Can you work these out from the model? Positions are in its coordinate system, mm. Face numbers are marked on the shaded views. A direction names the side the tool comes from. Give positions to 0.01 mm unless a question says otherwise; leave off trailing zeros. Order: outer loops, then holes, each group sorted by start corner. A loop starts at its lowest first (then second) coordinate and runs counter-clockwise, first axis right, second up. Notation, with made-up numbers: M -18,76.25 L 30,76.25 A35 ccw 30,109.25 Z; hole C 7,61 d4. An arc over 180 degrees is marked long. One line per question, with ' | ' between items. Start each with the question number.
1) If we section it at A-A, the plane z = -57: Please give me the cut outline in (x, y) (3 decimals).
2) For the marked faces 1 and 2, which set-ups out of +Z, -Z, +X, -X, +Y, -Y let a thin tool reach every point of the face, with its end or its side?
3) If we section it at C-C, the plane x = 33: Please give me the cut outline in (y, z) (3 decimals), plus the area to 3 significant figures.
4) Please list where these lines run through material, in increasing order: line 1 along X through (y, z) = (-46, -16); line 2 along Y through (x, z) = (29.5, -2) (3 decimals); line 3 along Z through (x, y) = (55.5, -19.5). Write a range as [from, to].
5) If we section it at B-B, the plane y = 160: Please give me the cut outline in (x, z).
6) If we section it at D-D, the plane y = -24: Please give me the cut outline in (x, z), plus the area to 3 significant figures.
7) I'm going to push flat-ended pins straight in: pin 1 Ø2 at (x, y) = (47.5, 255.5) entering from +Z; pin 2 Ø0.8 at (x, z) = (-48.5, -83) entering from -Y (3 decimals); pin 3 Ø10 at (y, z) = (-34.5, -48) entering from +X; pin 4 Ø1.2 at (x, z) = (-48, -7) entering from +Y (3 decimals). Where does each tip first touch, or does it pass through?
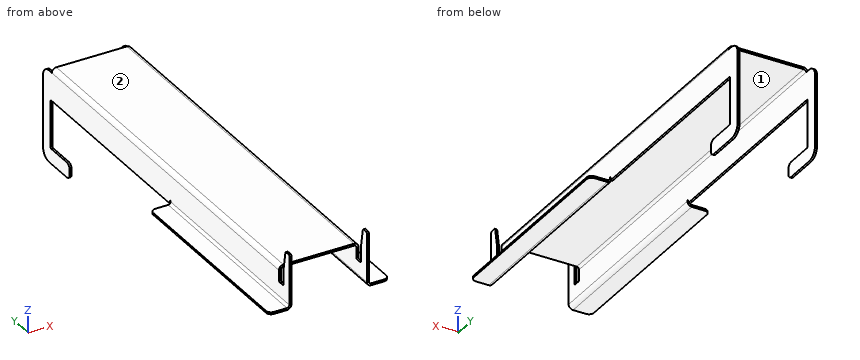
```python
from build123d import *

# Parameters (mm, degrees)
SKETCH1_W                     = 99.06
SKETCH1_H                     = 508
BASE_FLANGE1_DEPTH            = 2.5
EDGE_FLANGE1_STRIP_W          = 16
EDGE_FLANGE1_STRIP_H          = 2.5
EDGE_FLANGE1_STRIP_CUT_DEPTH  = 508
EDGE_FLANGE1_DEPTH            = 508
EDGE_FLANGE2_STRIP_W          = 16
EDGE_FLANGE2_STRIP_H          = 2.5
EDGE_FLANGE2_STRIP_CUT_DEPTH  = 254
EDGE_FLANGE2_RELIEF_W         = 17.25
EDGE_FLANGE2_RELIEF_H         = 1.25
EDGE_FLANGE2_RELIEF_CUT_DEPTH = 2.5
EDGE_FLANGE2_DEPTH            = 254
EDGE_FLANGE2_START            = 2.5
EDGE_FLANGE2_FLAT_DEPTH       = 2.5
EDGE_FLANGE3_STRIP_W          = 16
EDGE_FLANGE3_STRIP_H          = 2.5
EDGE_FLANGE3_STRIP_CUT_DEPTH  = 508
EDGE_FLANGE3_DEPTH            = 508
EDGE_FLANGE4_STRIP_W          = 16
EDGE_FLANGE4_STRIP_H          = 2.5
EDGE_FLANGE4_STRIP_CUT_DEPTH  = 254
EDGE_FLANGE4_RELIEF_W         = 17.25
EDGE_FLANGE4_RELIEF_H         = 1.25
EDGE_FLANGE4_RELIEF_CUT_DEPTH = 2.5
EDGE_FLANGE4_DEPTH            = 254
EDGE_FLANGE4_START            = 2.5
EDGE_FLANGE4_FLAT_DEPTH       = 2.5
SKETCH22_W                    = 5.5
SKETCH22_H                    = 22.225
CUT_EXTRUDE5_DEPTH            = 287.118684465
TAB1_DEPTH                    = 2.5
TAB2_START                    = -2.5
TAB2_DEPTH                    = 2.5
TAB3_DEPTH                    = 2.5
TAB4_START                    = -2.5
TAB4_DEPTH                    = 2.5
SKETCH47_W                    = 14.2875
SKETCH47_H                    = 9.525
CUT_EXTRUDE6_DEPTH            = 337.63035334
FILLET2_R                     = 1.5875
FILLET3_R                     = 1.5875
SKETCH48_W                    = 2.54
SKETCH48_H                    = 15.875
CUT_EXTRUDE9_DEPTH            = 337.63035334
FILLET4_R                     = 12.7


# Read off the part's stored shape, not the designer's step: Tab2
# Sheet-metal steps are written as plain solids
with BuildPart() as part:
    # Sketch1 → Base-Flange1 (new body)
    with BuildSketch(Plane.XY):
        Rectangle(SKETCH1_W, SKETCH1_H)
    extrude(amount=-BASE_FLANGE1_DEPTH)

    # Edge-Flange1 strip (across the edge) → Edge-Flange1 strip cut (cut)
    with BuildSketch(Plane(origin=(-49.53, -254, -2.5), x_dir=(1, 0, 0), z_dir=(0, 1, 0))):
        with Locations((-2.5, -1.25)):
            Rectangle(EDGE_FLANGE1_STRIP_W, EDGE_FLANGE1_STRIP_H)
    extrude(amount=EDGE_FLANGE1_STRIP_CUT_DEPTH, mode=Mode.SUBTRACT)

    # Edge-Flange1 section (across the edge) → Edge-Flange1 (add)
    with BuildSketch(Plane(origin=(-49.53, -254, -2.5), x_dir=(1, 0, 0), z_dir=(0, 1, 0))):
        with BuildLine():
            Line((0, 3), (0, 38.1))
            Line((0, 38.1), (2.5, 38.1))
            Line((2.5, 38.1), (2.5, 3))
            ThreePointArc((2.5, 3), (3.378679656, 0.878679656), (5.5, 0))
            Line((5.5, 0), (5.5, -2.5))
            ThreePointArc((5.5, -2.5), (1.610912703, -0.889087297), (0, 3))
        make_face()
    extrude(amount=EDGE_FLANGE1_DEPTH)

    # Edge-Flange2 strip (across the edge) → Edge-Flange2 strip cut (cut)
    with BuildSketch(Plane(origin=(-49.53, 0, -40.6), x_dir=(0, 0, 1), z_dir=(0, -1, 0))):
        with Locations((-5, -1.25)):
            Rectangle(EDGE_FLANGE2_STRIP_W, EDGE_FLANGE2_STRIP_H)
    extrude(amount=EDGE_FLANGE2_STRIP_CUT_DEPTH, mode=Mode.SUBTRACT)

    # Edge-Flange2 relief (on the sheet) → Edge-Flange2 relief cut (cut)
    with BuildSketch(Plane(origin=(-49.53, 0, -37.6), x_dir=(0, 0, 1), z_dir=(-1, 0, 0))):
        with Locations((-7.375, 0.625)):
            Rectangle(EDGE_FLANGE2_RELIEF_W, EDGE_FLANGE2_RELIEF_H)
    extrude(amount=-EDGE_FLANGE2_RELIEF_CUT_DEPTH, mode=Mode.SUBTRACT)

    # Edge-Flange2 bend section (across the edge) → Edge-Flange2 (add)
    with BuildSketch(Plane(origin=(-49.53, 0, -40.6), x_dir=(0, 0, 1), z_dir=(0, -1, 0))):
        with BuildLine():
            Line((-2.5, 3), (0, 3))
            ThreePointArc((0, 3), (0.878679656, 0.878679656), (3, 0))
            Line((3, 0), (3, -2.5))
            ThreePointArc((3, -2.5), (-0.889087297, -0.889087297), (-2.5, 3))
        make_face()
    extrude(amount=EDGE_FLANGE2_DEPTH)

    # Edge-Flange2 profile (on flange) → Edge-Flange2 flat (add)
    with BuildSketch(Plane(origin=(-49.53, 0, -40.6), x_dir=(0, -1, 0), z_dir=(0, 0, -1)).offset(EDGE_FLANGE2_START)):
        with BuildLine():
            Line((254, 3), (254, 19.05))
            ThreePointArc((254, 19.05), (252.140128061, 23.540128061), (247.65, 25.4))
            Line((247.65, 25.4), (6.35, 25.4))
            ThreePointArc((6.35, 25.4), (1.859871939, 23.540128061), (0, 19.05))
            Line((0, 19.05), (0, 3))
            Line((0, 3), (254, 3))
        make_face()
    extrude(amount=-EDGE_FLANGE2_FLAT_DEPTH)

    # Edge-Flange3 strip (across the edge) → Edge-Flange3 strip cut (cut)
    with BuildSketch(Plane(origin=(49.53, 254, -2.5), x_dir=(-1, 0, 0), z_dir=(0, -1, 0))):
        with Locations((-2.5, -1.25)):
            Rectangle(EDGE_FLANGE3_STRIP_W, EDGE_FLANGE3_STRIP_H)
    extrude(amount=EDGE_FLANGE3_STRIP_CUT_DEPTH, mode=Mode.SUBTRACT)

    # Edge-Flange3 section (across the edge) → Edge-Flange3 (add)
    with BuildSketch(Plane(origin=(49.53, 254, -2.5), x_dir=(-1, 0, 0), z_dir=(0, -1, 0))):
        with BuildLine():
            Line((0, 3), (0, 38.1))
            Line((0, 38.1), (2.5, 38.1))
            Line((2.5, 38.1), (2.5, 3))
            ThreePointArc((2.5, 3), (3.378679656, 0.878679656), (5.5, 0))
            Line((5.5, 0), (5.5, -2.5))
            ThreePointArc((5.5, -2.5), (1.610912703, -0.889087297), (0, 3))
        make_face()
    extrude(amount=EDGE_FLANGE3_DEPTH)

    # Edge-Flange4 strip (across the edge) → Edge-Flange4 strip cut (cut)
    with BuildSketch(Plane(origin=(49.53, -254, -40.6), x_dir=(0, 0, 1), z_dir=(0, 1, 0))):
        with Locations((-5, -1.25)):
            Rectangle(EDGE_FLANGE4_STRIP_W, EDGE_FLANGE4_STRIP_H)
    extrude(amount=EDGE_FLANGE4_STRIP_CUT_DEPTH, mode=Mode.SUBTRACT)

    # Edge-Flange4 relief (on the sheet) → Edge-Flange4 relief cut (cut)
    with BuildSketch(Plane(origin=(49.53, -254, -37.6), x_dir=(0, 0, 1), z_dir=(1, 0, 0))):
        with Locations((-7.375, -254.625)):
            Rectangle(EDGE_FLANGE4_RELIEF_W, EDGE_FLANGE4_RELIEF_H)
    extrude(amount=-EDGE_FLANGE4_RELIEF_CUT_DEPTH, mode=Mode.SUBTRACT)

    # Edge-Flange4 bend section (across the edge) → Edge-Flange4 (add)
    with BuildSketch(Plane(origin=(49.53, -254, -40.6), x_dir=(0, 0, 1), z_dir=(0, 1, 0))):
        with BuildLine():
            Line((-2.5, 3), (0, 3))
            ThreePointArc((0, 3), (0.878679656, 0.878679656), (3, 0))
            Line((3, 0), (3, -2.5))
            ThreePointArc((3, -2.5), (-0.889087297, -0.889087297), (-2.5, 3))
        make_face()
    extrude(amount=EDGE_FLANGE4_DEPTH)

    # Edge-Flange4 profile (on flange) → Edge-Flange4 flat (add)
    with BuildSketch(Plane(origin=(49.53, 0, -40.6), x_dir=(0, 1, 0), z_dir=(0, 0, -1)).offset(EDGE_FLANGE4_START)):
        with BuildLine():
            Line((-254, 19.05), (-254, 3))
            Line((-254, 3), (0, 3))
            Line((0, 3), (0, 19.05))
            ThreePointArc((0, 19.05), (-1.859871939, 23.540128061), (-6.35, 25.4))
            Line((-6.35, 25.4), (-247.65, 25.4))
            ThreePointArc((-247.65, 25.4), (-252.140128061, 23.540128061), (-254, 19.05))
        make_face()
    extrude(amount=-EDGE_FLANGE4_FLAT_DEPTH)

    # Sketch22 → Cut-Extrude5 (cut, through all)
    with BuildSketch(Plane.ZY.offset(49.53)):
        with Locations((-2.75, -242.8875)):
            Rectangle(SKETCH22_W, SKETCH22_H)
    extrude(amount=-CUT_EXTRUDE5_DEPTH, mode=Mode.SUBTRACT)

    # Sketch30 → Tab1 (add)
    with BuildSketch(Plane.ZY.offset(49.53)):
        Polygon((-5.5, -254), (24.6625, -254), (24.6625, -245.77870531), (-0.7375, -241.3), (-5.5, -241.3), align=None)
    extrude(amount=-TAB1_DEPTH)

    # Tab2 outline → Tab2 (add)
    with BuildSketch(Plane(origin=(49.53, 0, 0), x_dir=(0, 0, -1), z_dir=(1, 0, 0)).offset(TAB2_START)):
        Polygon((-24.6625, -254), (5.5, -254), (5.5, -241.3), (0.7375, -241.3), (-24.6625, -245.77870531), align=None)
    extrude(amount=TAB2_DEPTH)

    # Sketch43 → Tab3 (add)
    with BuildSketch(Plane(origin=(49.53, 0, 0), x_dir=(0, 0, -1), z_dir=(1, 0, 0))):
        with BuildLine():
            Line((8.675031572, 288.925), (116.625031572, 288.925))
            ThreePointArc((116.625031572, 288.925), (118.870095602, 287.99506403), (119.800031572, 285.75))
            Line((119.800031572, 285.75), (119.800031572, 254))
            Line((119.800031572, 254), (119.800031572, 222.25))
            ThreePointArc((119.800031572, 222.25), (117.940159632, 217.759871939), (113.450031572, 215.9))
            Line((113.450031572, 215.9), (107.100031572, 215.9))
            ThreePointArc((107.100031572, 215.9), (102.609903511, 217.759871939), (100.750031572, 222.25))
            Line((100.750031572, 222.25), (100.750031572, 250.825))
            Line((100.750031572, 250.825), (100.750031572, 254))
            Line((100.750031572, 254), (100.750031572, 255.5875))
            ThreePointArc((100.750031572, 255.5875), (100.285063587, 256.710032015), (99.162531572, 257.175))
            Line((99.162531572, 257.175), (42.1875, 257.175))
            ThreePointArc((42.1875, 257.175), (41.064967985, 256.710032015), (40.6, 255.5875))
            Line((40.6, 255.5875), (40.6, 254))
            Line((40.6, 254), (5.500031572, 254))
            Line((5.500031572, 254), (5.500031572, 285.75))
            ThreePointArc((5.500031572, 285.75), (6.429967542, 287.99506403), (8.675031572, 288.925))
        make_face()
    extrude(amount=-TAB3_DEPTH)

    # Sketch46 → Tab4 (add)
    with BuildSketch(Plane.ZY.offset(49.53).offset(TAB4_START)):
        with BuildLine():
            Line((-116.625, 288.925), (-8.675, 288.925))
            ThreePointArc((-8.675, 288.925), (-6.42993597, 287.99506403), (-5.5, 285.75))
            Line((-5.5, 285.75), (-5.5, 254))
            Line((-5.5, 254), (-40.6, 254))
            Line((-40.6, 254), (-40.6, 255.5875))
            ThreePointArc((-40.6, 255.5875), (-41.064967985, 256.710032015), (-42.1875, 257.175))
            Line((-42.1875, 257.175), (-99.458781194, 257.175))
            ThreePointArc((-99.458781194, 257.175), (-100.581313209, 256.710032015), (-101.046281194, 255.5875))
            Line((-101.046281194, 255.5875), (-101.046281194, 254))
            Line((-101.046281194, 254), (-101.046281194, 222.25))
            ThreePointArc((-101.046281194, 222.25), (-102.906153133, 217.759871939), (-107.396281194, 215.9))
            Line((-107.396281194, 215.9), (-113.45, 215.9))
            ThreePointArc((-113.45, 215.9), (-117.940128061, 217.759871939), (-119.8, 222.25))
            Line((-119.8, 222.25), (-119.8, 254))
            Line((-119.8, 254), (-119.8, 285.75))
            ThreePointArc((-119.8, 285.75), (-118.87006403, 287.99506403), (-116.625, 288.925))
        make_face()
    extrude(amount=TAB4_DEPTH)

    # Sketch47 → Cut-Extrude6 (cut, through all)
    with BuildSketch(Plane.ZY.offset(49.53)):
        with Locations((-12.64375, -236.5375)):
            Rectangle(SKETCH47_W, SKETCH47_H)
    extrude(amount=-CUT_EXTRUDE6_DEPTH, mode=Mode.SUBTRACT)

    # Fillet2
    fillet2_edges = [part.edges().sort_by_distance(p)[0] for p in [
        (48.28, -231.775, -19.7875),
        (48.28, -241.3, -19.7875),
        (-48.28, -231.775, -19.7875),
        (-48.28, -241.3, -19.7875),
    ]]
    fillet(fillet2_edges, radius=FILLET2_R)

    # Fillet3
    fillet3_edges = [part.edges().sort_by_distance(p)[0] for p in [
        (-48.28, -241.3, -0.7375),
        (-48.28, -245.77870531, 24.6625),
        (-48.28, -254, 24.6625),
        (48.28, -254, 24.6625),
        (48.28, -245.77870531, 24.6625),
        (48.28, -241.3, -0.7375),
    ]]
    fillet(fillet3_edges, radius=FILLET3_R)

    # Sketch48 → Cut-Extrude9 (cut, through all)
    with BuildSketch(Plane.ZY.offset(49.53)):
        with BuildLine():
            Line((-8.675, 288.925), (-116.625, 288.925))
            ThreePointArc((-116.625, 288.925), (-118.87006403, 287.99506403), (-119.8, 285.75))
            Line((-119.8, 285.75), (-119.8, 273.05))
            Line((-119.8, 273.05), (-5.5, 273.05))
            Line((-5.5, 273.05), (-5.5, 285.75))
            ThreePointArc((-5.5, 285.75), (-6.42993597, 287.99506403), (-8.675, 288.925))
        make_face()
        with Locations((-121.07, 280.9875)):
            Rectangle(SKETCH48_W, SKETCH48_H)
    extrude(amount=-CUT_EXTRUDE9_DEPTH, mode=Mode.SUBTRACT)


with BuildPart() as cut_extrude9_kept_piece:
    # of the separate pieces the step leaves, the one the design keeps (cut_extrude9_pieces_kept)
    add(part.part.solids().sort_by_distance((47.03, -241.3, -0.876388253))[0])

    # Fillet4
    fillet4_edges = [cut_extrude9_kept_piece.edges().sort_by_distance(p)[0] for p in [
        (-48.28, 273.05, -119.8),
        (48.28, 273.05, -5.500031572),
        (48.28, 273.05, -119.800031572),
        (-48.28, 273.05, -5.5),
    ]]
    fillet(fillet4_edges, radius=FILLET4_R)


solid = cut_extrude9_kept_piece.part
```
Results found:
1) outline: M -49.53,257.175 L -47.03,257.175 L -47.03,273.05 L -49.53,273.05 Z; M 47.03,257.175 L 49.53,257.175 L 49.53,273.05 L 47.03,273.05 Z
2) face 1: -Z, +Y, -Y | face 2: +Z, +X, -X, +Y, -Y
3) outline: M -231.775,-2.5 L 254,-2.5 L 254,0 L -231.775,0 Z | area: 1,210 mm²
4) line 1: x = [-49.53, -47.03], [47.03, 49.53] | line 2: y = [-231.775, 254] | line 3: z = [-43.1, -40.6]
5) outline: M -49.53,-40.6 L -47.03,-40.6 L -47.03,-5.5 A3 cw -44.03,-2.5 L 44.03,-2.5 A3 cw 47.03,-5.5 L 47.03,-40.6 L 49.53,-40.6 L 49.53,-5.5 A5.5 ccw 44.03,0 L -44.03,0 A5.5 ccw -49.53,-5.5 Z
6) outline: M -74.93,-43.1 L -52.53,-43.1 A5.5 ccw -47.03,-37.6 L -47.03,-5.5 A3 cw -44.03,-2.5 L 44.03,-2.5 A3 cw 47.03,-5.5 L 47.03,-37.6 A5.5 ccw 52.53,-43.1 L 74.93,-43.1 L 74.93,-40.6 L 52.53,-40.6 A3 cw 49.53,-37.6 L 49.53,-5.5 A5.5 ccw 44.03,0 L -44.03,0 A5.5 ccw -49.53,-5.5 L -49.53,-37.6 A3 cw -52.53,-40.6 L -74.93,-40.6 Z | area: 559 mm²
7) pin 1: stops at z = -5.5 | pin 2: stops at y = 257.175 | pin 3: stops at x = 74.93 | pin 4: stops at y = 267.345
